Check sheet for the modelled part. Datum: model origin and axes. Units: mm. A direction names the side the tool comes from. Coordinates: 2 decimals unless noted, no trailing zeros. Write each loop counter-clockwise with the first axis right and the second up, starting at its lowest first coordinate (ties: lowest second). Pieces come first, ordered by that corner, then holes. Notation, with made-up numbers: (-33, 36.5) - (-29, 36.5) arc R18 ccw to (-29, 66.5) - close; hole circle Ø10 at (-32.5, -25). An arc over 180 degrees is marked (long way). Use one line per item in the form item = value. Start each with the question number.
1. Cross-section at D-D on x = -5. Record the boundary of the cut face in (y, z).
2. Scan lines: line 1 along X through (y, z) = (0, 2.65); line 2 along Z through (x, y) = (-4.25, 3.25). Record each from-to range of solid material in increasing order.
3. Cross-section at C-C on z = 2.95. Record the boundary of the cut face in (x, y).
4. Draft check along Y on faces 5 (the face through (-1, -4, 0)), 6 (the face through (-4.197, -1.322, 3.728)), 7 (the face through (2.81, -1.63, 5.11)). Enter one of: +Y half, -Y half, draft (parallel to the pull), parting line (faces both ways), or undercut.
5. Tool access check on faces 1 (the face through (0.01, 3.25, 5.09)), 2 (the face through (-3.434, -1.081, 2.825)), 3 (the face through (1.535, 2.634, 5.346)), 4 (the face through (-4.197, -1.322, 0.177)). Record the directions out of +Z, -Z, +X, -X, +Y, -Y that give a thin tool (end or side, any length) a straight path to the whole face; none if there is none.
6. Go/stop test with flat-tipped pins: pin 1 Ø2 at (x, z) = (4, 3.5) entering from -Y; pin 2 Ø4.5 at (x, y) = (0, 0) entering from +Z; pin 3 Ø2 at (y, z) = (-4.5, 3.5) entering from +X; pin 4 Ø1 at (y, z) = (0.5, 2.5) entering from -X. Record where each tip stops, or that it passes through.
```python
from build123d import *

# Parameters (mm, degrees)
POCKET_DEPTH       = 34.402163
POCKET_DEPTH_BACK  = 40.002163
POLARPATTERN_COUNT = 6


with BuildPart() as part:
    # Sketch → Revolution (revolve)
    with BuildSketch(Plane.XZ):
        Polygon((-3.6, 4.6), (-3.6, 3.5), (-3.6, 2.5), (-3.6, 1), (-3.325, 0.5), (-3.825, 0), (-4.4, 0), (-4.4, 0.35), (-5.75, 0.35), (-5.75, 1), (-4.675, 1), (-4.675, 2.3), (-4.4, 2.575), (-4.4, 4.85), (-3.65, 5.6), (-3.15, 5.6), (-2.95, 5.1), (-3.15, 4.6), align=None)
    revolve(axis=Axis((0, 0, 0), (0, 0, 1)))

    # Sketch001 → Pocket (cut, two sides)
    with BuildSketch(Plane.XY) as pocket_sk:
        with BuildLine():
            Line((0, 0), (-0.776457, 2.897777))
            ThreePointArc((-0.587735, 3.196415), (-0.747472, 3.08841), (-0.776457, 2.897777))
            ThreePointArc((0.587735, 3.196415), (0, 3.25), (-0.587735, 3.196415))
            ThreePointArc((0.776457, 2.897777), (0.747472, 3.08841), (0.587735, 3.196415))
            Line((0.776457, 2.897777), (0, 0))
        make_face()
    pocket = extrude(amount=-POCKET_DEPTH, mode=Mode.SUBTRACT) + extrude(pocket_sk.sketch, amount=POCKET_DEPTH_BACK, mode=Mode.SUBTRACT)

    # PolarPattern: Pocket ×6 about axis
    polarpattern_axis = Axis((0, 0, 0), (0, 0, 1))
    for i in range(1, POLARPATTERN_COUNT):
        add(pocket.rotate(polarpattern_axis, i * 360 / POLARPATTERN_COUNT), mode=Mode.SUBTRACT)


solid = part.part
```
Final values:
q1.outline = (-2.84, 0.35) - (2.84, 0.35) - (2.84, 1) - (-2.84, 1) - close
q2.line_1 = -4.4 to -3.6, 3.6 to 4.4
q2.line_2 = 0.35 to 1
q3.outline = circle Ø8.8 at (0, 0); hole circle Ø7.2 at (0, 0)
q4.face_5 = draft
q4.face_6 = parting line
q4.face_7 = undercut
q5.face_1 = +Z, -Z
q5.face_2 = none
q5.face_3 = +Z
q5.face_4 = -Z
q6.pin_1 = -3.22
q6.pin_2 = through
q6.pin_3 = 2.67
q6.pin_4 = -4.67
